The listing builds one solid part. Answer for the finished solid, in the listing's coordinates (mm). A direction names the side the tool comes from. Give positions to 0.01 mm unless a question says otherwise; leave off trailing zeros. Loops run counter-clockwise (first coordinate to the right, second up) from the corner with the lowest first, then second, coordinate; pieces in that order, holes last. Notation, with made-up numbers: M 72,47 L 88,47 A31 cw 88,81 Z; hole C 78.25,27.5 d9. An arc over 180 degrees is marked long. Return JSON: item names as keys, results as strings.
from build123d import *

# Parameters (mm, degrees)
BOX002_W          = 36
BOX002_H          = 16
BOX002_DEPTH      = 41
CYLINDER035_R     = 13
CYLINDER035_DEPTH = 24
CYLINDER003_R     = 1.5
CYLINDER003_DEPTH = 44
CYLINDER002_R     = 1.5
CYLINDER002_DEPTH = 44
PAD009_DEPTH      = 50
SKETCH026_W       = 10
SKETCH026_H       = 27
POCKET006_DEPTH   = 38


with BuildPart() as cubo002:
    # Box002 → Box002 (new body)
    with BuildSketch(Plane(origin=(-19, 1, 45), x_dir=(1, 0, 0), z_dir=(0, 0, 1))):
        with Locations((18, 8)):
            Rectangle(BOX002_W, BOX002_H)
    extrude(amount=BOX002_DEPTH)


with BuildPart() as cut013020:
    # Cylinder035 → Cylinder035 (new body)
    with BuildSketch(Plane(origin=(0, 17, 45), x_dir=(1, 0, 0), z_dir=(0, 0, 1))):
        Circle(CYLINDER035_R)
    extrude(amount=CYLINDER035_DEPTH)

    # Cut013020: cut Cubo002
    add(cubo002.part, mode=Mode.SUBTRACT)


with BuildPart() as cut013020_1:
    # Cut013020 placement: moved
    add(cut013020.part.moved(Location((0, 3, -14))))


with BuildPart() as cilindro003:
    # Cylinder003 → Cylinder003 (new body)
    with BuildSketch(Plane(origin=(17, 63, -20), x_dir=(1, 0, 0), z_dir=(0, 0, 1))):
        Circle(CYLINDER003_R)
    extrude(amount=CYLINDER003_DEPTH)


with BuildPart() as fusion001009:
    # Cylinder002 → Cylinder002 (new body)
    with BuildSketch(Plane(origin=(-17, 63, -22), x_dir=(1, 0, 0), z_dir=(0, 0, 1))):
        Circle(CYLINDER002_R)
    extrude(amount=CYLINDER002_DEPTH)

    # Fusion001009: union Cilindro003
    add(cilindro003.part)


with BuildPart() as fusion001009_1:
    # Fusion001009 placement: moved
    add(fusion001009.part.moved(Location((0, -15, 0))))


with BuildPart() as cut013021:
    # Sketch014 → Pad009 (new body)
    with BuildSketch(Plane.YZ):
        Polygon((-20, -7.5), (-20, 18), (20, 18), (20, 2.5), (10, 2.5), (10, -2.5), (20, -2.5), (20, -7.5), align=None)
    extrude(amount=PAD009_DEPTH)

    # Sketch026 (on Face3 of Pad009) → Pocket006 (cut)
    with BuildSketch(Plane.ZX.offset(20)):
        with Locations((10.160879, 25.010977)):
            Rectangle(SKETCH026_W, SKETCH026_H)
    extrude(amount=-POCKET006_DEPTH, mode=Mode.SUBTRACT)


with BuildPart() as cut013021_1:
    # Body013 placement: moved
    add(cut013021.part.moved(Location((-25, 31, -5))))

    # Cut013018: cut Fusion001009
    add(fusion001009_1.part, mode=Mode.SUBTRACT)


with BuildPart() as cut013021_2:
    # Cut013018 placement: moved
    add(cut013021_1.part.moved(Location((0, 8, 31))))

    # Cut013021: cut Cut013020
    add(cut013020_1.part, mode=Mode.SUBTRACT)


solid = cut013021_2.part
(1) Given pin 1 (1.8 mm diameter, centred on x = 17, y = 56, fed in from +Z); pin 2 (1.5 mm diameter, centred on x = 12.5, z = 32, fed in from +Y); pin 3 (2 mm diameter, centred on x = -3.5, z = 33.5, fed in from +Y), each flat-ended and moving along its own axis, determine where each tip first touches the part or whether it passes through.
Values follow:
{"pin 1": "through", "pin 2": "y = 21", "pin 3": "y = 20"}
(2) A tool of negligible diameter and unlimited length cuts with its end or side. For faces 4 (the flat face through (-13.489, 40, 36)), 5 (the flat face through (0, 54, 28.5)), 6 (the cylindrical face through (15.5, 56.07, 36.14)), 7 (the flat face through (0, 25, 31)), from which of +Z, -Z, +X, -X, +Y, -Y can it reach the whole face along a straight path? Write none if from no direction.
Values follow:
{"face 4": "+Y", "face 5": "+X, -X, +Y", "face 6": "+Z, -Z", "face 7": "+Z"}
(3) Straight lines are drawn through the part: line 1 along Z through (x, y) = (0.5, 49.5); line 2 along X through (y, z) = (56, 22.4); line 3 along Z through (x, y) = (-1, 40.5). For each, find the intervals that lie inside material, in ascending order.
Values follow:
{"line 1": "18.5 to 23.5, 28.5 to 31.16, 41.16 to 44", "line 2": "-25 to -18.5, -15.5 to 15.5, 18.5 to 25", "line 3": "18.5 to 31.16, 41.16 to 44"}
(4) The part is cut by section B-B (y = 50). Determine the outline of the cut face in (x, z), and give its area (3 significant figures).
Values follow:
{"outline": "M -25,18.5 L 25,18.5 L 25,23.5 L -25,23.5 Z; M -25,28.5 L 25,28.5 L 25,44 L -25,44 Z; hole M -13.49,31.16 L 13.51,31.16 L 13.51,41.16 L -13.49,41.16 Z", "area": "755 mm²"}
(5) The part is cut by section D-D (z = 36.5). Determine the outline of the cut face in (x, y).
Values follow:
{"outline": "M -25,19 L 25,19 L 25,59 L 13.51,59 L 13.51,21 L 12.96,21 A13 cw 13,20 L -13,20 A13 cw -12.96,21 L -13.49,21 L -13.49,59 L -25,59 Z; hole C -17,56 d3; hole C 17,56 d3"}
(6) The part is cut by section C-C (x = 17). Determine the outline of the cut face in (y, z), and give its area (4 significant figures).
Values follow:
{"outline": "M 19,18.5 L 54.5,18.5 L 54.5,23.5 L 49,23.5 L 49,28.5 L 54.5,28.5 L 54.5,44 L 19,44 Z; M 57.5,18.5 L 59,18.5 L 59,23.5 L 57.5,23.5 Z; M 57.5,28.5 L 59,28.5 L 59,44 L 57.5,44 Z", "area": "908.5 mm²"}
(7) The part is cut by section A-A (y = 56). Determine the outline of the cut face in (x, z), and give its area (3 significant figures).
Values follow:
{"outline": "M -25,18.5 L -18.5,18.5 L -18.5,23.5 L -25,23.5 Z; M -25,28.5 L -18.5,28.5 L -18.5,44 L -25,44 Z; M -15.5,18.5 L 15.5,18.5 L 15.5,23.5 L -15.5,23.5 Z; M -15.5,28.5 L 15.5,28.5 L 15.5,44 L -15.5,44 Z; M 18.5,18.5 L 25,18.5 L 25,23.5 L 18.5,23.5 Z; M 18.5,28.5 L 25,28.5 L 25,44 L 18.5,44 Z; hole M -13.49,31.16 L 13.51,31.16 L 13.51,41.16 L -13.49,41.16 Z", "area": "632 mm²"}
(8) Determine the mould class of faces 1 (the cylindrical face through (-18.5, 56.07, 20.96)), 2 (the flat face through (-25, 39, 31)), 3 (the flat face through (0, 59, 42)) for opening direction Y: released by +Y, released by -Y, zero draft, split by the parting line, or undercut.
Values follow:
{"face 1": "undercut", "face 2": "zero draft", "face 3": "released by +Y"}
